For this review, take the finished solid that the model builds, in its own axes (mm). A direction names the side the tool comes from. Coordinates: 2 decimals unless noted, no trailing zeros. Loops run counter-clockwise (first coordinate to the right, second up) from the corner with the lowest first, then second, coordinate; pieces in that order, holes last. Notation, with made-up numbers: M -8,51.5 L 38,51.5 A9 cw 38,67.5 Z; hole C -28,30.25 d8. An arc over 180 degrees is marked long. Put each result on its own line as item: value.
```python
from build123d import *

# Parameters (mm, degrees)
SKETCH1_W               = 50
SKETCH1_H               = 51
BOSS_EXTRUDE1_DEPTH     = 3
SKETCH2_W               = 50
SKETCH2_H               = 3
BOSS_EXTRUDE2_DEPTH     = 50
FILLET1_R               = 2
CHAMFER1_SIZE           = 5
SKETCH4_R               = 12.55
SKETCH4_R_2             = 2.1
CUT_EXTRUDE2_DEPTH      = 50
BOSS_EXTRUDE3_DEPTH     = 3
CROQUIS1_W              = 117.155
CROQUIS1_H              = 77.15
SALIENTE_EXTRUIR1_DEPTH = 10
CROQUIS2_W              = 76.4
CROQUIS2_H              = 56.4
SALIENTE_EXTRUIR2_DEPTH = 7.5
CROQUIS3_R              = 2
CORTAR_EXTRUIR1_DEPTH   = 27.5
CROQUIS4_W              = 91
CROQUIS4_H              = 72
CROQUIS4_W_2            = 79
CROQUIS4_H_2            = 57
SALIENTE_EXTRUIR3_DEPTH = 120
CUT_EXTRUDE1_DEPTH      = 50
CROQUIS5_W              = 66
CROQUIS5_H              = 90
CORTAR_EXTRUIR2_DEPTH   = 64
CROQUIS7_R              = 2.1
CORTAR_EXTRUIR3_DEPTH   = 20
CROQUIS9_R              = 2
CORTAR_EXTRUIR5_DEPTH   = 110
CROQUIS8_R              = 2
CORTAR_EXTRUIR6_DEPTH   = 120
CROQUIS10_R             = 17.5
SALIENTE_EXTRUIR4_DEPTH = 7.5
CROQUIS11_W             = 81
CROQUIS11_H             = 10
CROQUIS11_W_2           = 5
CORTAR_EXTRUIR7_DEPTH   = 7.9
CROQUIS12_W             = 79
CROQUIS12_H             = 4.5
SALIENTE_EXTRUIR5_DEPTH = 12.5
CROQUIS14_W             = 10
CROQUIS14_H             = 3.6
CORTAR_EXTRUIR8_DEPTH   = 100
CROQUIS21_R             = 1.25
CORTAR_EXTRUIR10_DEPTH  = 4
CROQUIS22_R             = 1.5
CORTAR_EXTRUIR11_DEPTH  = 40
CROQUIS23_W             = 10
CROQUIS23_H             = 10
CORTAR_EXTRUIR12_DEPTH  = 10
CROQUIS24_W             = 2
CROQUIS24_H             = 52.5
CORTAR_EXTRUIR13_DEPTH  = 22.5


with BuildPart() as part:
    # Sketch1 → Boss-Extrude1 (new body)
    with BuildSketch(Plane.XY):
        Rectangle(SKETCH1_W, SKETCH1_H)
    extrude(amount=BOSS_EXTRUDE1_DEPTH)

    # Sketch2 → Boss-Extrude2 (add)
    with BuildSketch(Plane.XY.offset(3)):
        with Locations((0, -24)):
            Rectangle(SKETCH2_W, SKETCH2_H)
    extrude(amount=BOSS_EXTRUDE2_DEPTH)

    # Fillet1
    fillet1_edges = [part.edges().sort_by_distance(p)[0] for p in [
        (0, -22.5, 3),
        (0, -25.5, 0),
    ]]
    fillet(fillet1_edges, radius=FILLET1_R)

    # Chamfer1
    chamfer1_edges = [part.edges().sort_by_distance(p)[0] for p in [
        (-25, -24, 53),
        (25, -24, 53),
        (-25, 25.5, 1.5),
        (25, 25.5, 1.5),
    ]]
    chamfer(chamfer1_edges, length=CHAMFER1_SIZE)

    # Sketch4 → Cut-Extrude2 (cut)
    with BuildSketch(Plane.XY.offset(3)):
        with Locations((0, 4.5)):
            Circle(SKETCH4_R)
        with Locations((0, 22)):
            Circle(SKETCH4_R_2)
        with Locations((0, -13)):
            Circle(SKETCH4_R_2)
        with Locations((17.5, 4.5)):
            Circle(SKETCH4_R_2)
        with Locations((-17.5, 4.5)):
            Circle(SKETCH4_R_2)
    extrude(amount=-CUT_EXTRUDE2_DEPTH, mode=Mode.SUBTRACT)

    # Sketch5 → Boss-Extrude3 (add)
    with BuildSketch(Plane.ZY.offset(25)):
        with BuildLine():
            Line((3, -2.5), (16, -22.5))
            Line((16, -22.5), (5, -22.5))
            ThreePointArc((5, -22.5), (3.585786438, -21.914213562), (3, -20.5))
            Line((3, -20.5), (3, -2.5))
        make_face()
    boss_extrude3 = extrude(amount=-BOSS_EXTRUDE3_DEPTH)

    # Mirror1: Boss-Extrude3 across plane
    add(boss_extrude3.mirror(Plane(origin=(0, 0, 0), x_dir=(0, 0, 1), z_dir=(1, 0, 0))))



with BuildPart() as body_2:
    # Croquis1 → Saliente-Extruir1 (new body)
    with BuildSketch(Plane(origin=(0, 0, 55), x_dir=(-1, 0, 0), z_dir=(0, 0, -1))):
        with Locations((0.0025, 0)):
            Rectangle(CROQUIS1_W, CROQUIS1_H)
    extrude(amount=-SALIENTE_EXTRUIR1_DEPTH)

    # Croquis2 → Saliente-Extruir2 (add)
    with BuildSketch(Plane.XY.offset(65)):
        Rectangle(CROQUIS2_W, CROQUIS2_H)
    extrude(amount=SALIENTE_EXTRUIR2_DEPTH)

    # Croquis3 → Cortar-Extruir1 (cut)
    with BuildSketch(Plane(origin=(0, 0, 55), x_dir=(-1, 0, 0), z_dir=(0, 0, -1))):
        with Locations((50.58, -18.575)):
            Circle(CROQUIS3_R)
        with Locations((50.58, 18.575)):
            Circle(CROQUIS3_R)
    cortar_extruir1 = extrude(amount=-CORTAR_EXTRUIR1_DEPTH, mode=Mode.SUBTRACT)

    # Simetría1: Cortar-Extruir1 across plane
    add(cortar_extruir1.mirror(Plane(origin=(0, 0, 0), x_dir=(0, 0, 1), z_dir=(1, 0, 0))), mode=Mode.SUBTRACT)


with BuildPart() as part_1:
    add(part.part)

    add(body_2.part)  # Saliente-Extruir3 merges body 2
    # Croquis4 → Saliente-Extruir3 (add)
    with BuildSketch(Plane(origin=(0, 0, 55), x_dir=(-1, 0, 0), z_dir=(0, 0, -1))):
        with Locations((0.5, 2.5)):
            Rectangle(CROQUIS4_W, CROQUIS4_H)
        with Locations((1.5, 3)):
            Rectangle(CROQUIS4_W_2, CROQUIS4_H_2, mode=Mode.SUBTRACT)
    extrude(amount=SALIENTE_EXTRUIR3_DEPTH)

    # Sketch3 → Cut-Extrude1 (cut)
    with BuildSketch(Plane(origin=(0, -22.5, 0), x_dir=(1, 0, 0), z_dir=(0, 1, 0))):
        with BuildLine():
            Line((-17.1, -38), (-17.1, -37.9))
            ThreePointArc((-17.1, -37.9), (-15, -35.8), (-12.9, -37.9))
            Line((-12.9, -37.9), (-12.9, -38))
            ThreePointArc((-12.9, -38), (-15, -40.1), (-17.1, -38))
        make_face()
        with BuildLine():
            Line((12.9, -38), (12.9, -37.9))
            ThreePointArc((12.9, -37.9), (15, -35.8), (17.1, -37.9))
            Line((17.1, -37.9), (17.1, -38))
            ThreePointArc((17.1, -38), (15, -40.1), (12.9, -38))
        make_face()
    extrude(amount=-CUT_EXTRUDE1_DEPTH, mode=Mode.SUBTRACT)

    # Croquis5 → Cortar-Extruir2 (cut)
    with BuildSketch(Plane(origin=(0, 38.5, 0), x_dir=(1, 0, 0), z_dir=(0, 1, 0))):
        with Locations((-0.5, -10)):
            Rectangle(CROQUIS5_W, CROQUIS5_H)
    extrude(amount=-CORTAR_EXTRUIR2_DEPTH, mode=Mode.SUBTRACT)

    # Croquis7 → Cortar-Extruir3 (cut)
    with BuildSketch(Plane.XZ.offset(33.5)):
        with Locations((15, 19.753839811)):
            Circle(CROQUIS7_R)
        with Locations((-15, 19.753839811)):
            Circle(CROQUIS7_R)
    extrude(amount=-CORTAR_EXTRUIR3_DEPTH, mode=Mode.SUBTRACT)

    # Croquis9 → Cortar-Extruir5 (cut)
    with BuildSketch(Plane.ZY.offset(46)):
        with Locations((-49, -18.5)):
            Circle(CROQUIS9_R)
        with Locations((-49, 5.5)):
            Circle(CROQUIS9_R)
    extrude(amount=-CORTAR_EXTRUIR5_DEPTH, mode=Mode.SUBTRACT)

    # Croquis8 → Cortar-Extruir6 (cut)
    with BuildSketch(Plane(origin=(0, 38.5, 0), x_dir=(1, 0, 0), z_dir=(0, 1, 0))):
        with Locations((-10.5, 49)):
            Circle(CROQUIS8_R)
        with Locations((9.5, 49)):
            Circle(CROQUIS8_R)
    extrude(amount=-CORTAR_EXTRUIR6_DEPTH, mode=Mode.SUBTRACT)

    # Croquis10 → Saliente-Extruir4 (add)
    with BuildSketch(Plane(origin=(0, 0, -35), x_dir=(-1, 0, 0), z_dir=(0, 0, -1))):
        Polygon((41, 0), (41, -25.5), (-40, -25.5), (-40, 31.5), (41, 31.5), align=None)
        with Locations((0, 3)):
            Circle(CROQUIS10_R, mode=Mode.SUBTRACT)
    extrude(amount=SALIENTE_EXTRUIR4_DEPTH)

    # Croquis11 → Cortar-Extruir7 (cut)
    with BuildSketch(Plane(origin=(0, 38.5, 0), x_dir=(1, 0, 0), z_dir=(0, 1, 0))):
        with Locations((-0.5, 60)):
            Rectangle(CROQUIS11_W, CROQUIS11_H)
        with Locations((-43.5, 60)):
            Rectangle(CROQUIS11_W_2, CROQUIS11_H)
        with Locations((42.5, 60)):
            Rectangle(CROQUIS11_W_2, CROQUIS11_H)
    extrude(amount=-CORTAR_EXTRUIR7_DEPTH, mode=Mode.SUBTRACT)

    # Croquis12 → Saliente-Extruir5 (add)
    with BuildSketch(Plane(origin=(0, 0, -42.5), x_dir=(-1, 0, 0), z_dir=(0, 0, -1))):
        with Locations((1.5, 29.25)):
            Rectangle(CROQUIS12_W, CROQUIS12_H)
    extrude(amount=SALIENTE_EXTRUIR5_DEPTH)

    # Croquis14 → Cortar-Extruir8 (cut)
    with BuildSketch(Plane(origin=(45, 0, 0), x_dir=(0, 0, -1), z_dir=(1, 0, 0))):
        with Locations((60, 28.8)):
            Rectangle(CROQUIS14_W, CROQUIS14_H)
    extrude(amount=-CORTAR_EXTRUIR8_DEPTH, mode=Mode.SUBTRACT)

    # Croquis21 → Cortar-Extruir10 (cut)
    with BuildSketch(Plane(origin=(45, 0, 0), x_dir=(0, 0, -1), z_dir=(1, 0, 0))):
        with Locations((-40, 32)):
            Circle(CROQUIS21_R)
        with Locations((-40, 19)):
            Circle(CROQUIS21_R)
    extrude(amount=-CORTAR_EXTRUIR10_DEPTH, mode=Mode.SUBTRACT)

    # Croquis22 → Cortar-Extruir11 (cut)
    with BuildSketch(Plane.XZ.offset(33.5)):
        with Locations((30, -30)):
            Circle(CROQUIS22_R)
        with Locations((30, -20)):
            Circle(CROQUIS22_R)
    extrude(amount=-CORTAR_EXTRUIR11_DEPTH, mode=Mode.SUBTRACT)

    # Croquis23 → Cortar-Extruir12 (cut)
    with BuildSketch(Plane.ZY.offset(46)):
        with Locations((50, 8.5)):
            Rectangle(CROQUIS23_W, CROQUIS23_H)
    extrude(amount=-CORTAR_EXTRUIR12_DEPTH, mode=Mode.SUBTRACT)

    # Croquis24 → Cortar-Extruir13 (cut)
    with BuildSketch(Plane(origin=(0, 0, -65), x_dir=(-1, 0, 0), z_dir=(0, 0, -1))):
        with Locations((-39, 0.75)):
            Rectangle(CROQUIS24_W, CROQUIS24_H)
    extrude(amount=-CORTAR_EXTRUIR13_DEPTH, mode=Mode.SUBTRACT)


solid = part_1.part
```
(1) Add section A-A (z = 48.5). Write out the cut boundary in (x, y), plus the area to 3 significant figures.
Determined:
outline: M -46,-33.5 L 45,-33.5 L 45,38.5 L 32.5,38.5 L 32.5,31.5 L 38,31.5 L 38,-25.5 L -41,-25.5 L -41,3.5 L -46,3.5 Z; M -46,13.5 L -41,13.5 L -41,31.5 L -33.5,31.5 L -33.5,38.5 L -46,38.5 Z
area: 1,540 mm^2
(2) Draft analysis for pull direction Z (two halves, no side actions). For faces 4 (the flat face through (35, 31.5, 11)), 5 (the flat face through (40, 0, -54)), 6 (the flat face through (6, -28, -65)), state which applies: +Z half, -Z half, draft (parallel to the pull), parting line (faces both ways), or undercut.
Determined:
face 4: undercut
face 5: draft
face 6: -Z half
(3) Add section B-B (x = -36.5). Write out the cut boundary in (y, z) (3 decimals), plus the area to 3 significant figures.
Determined:
outline: M -38.575,55 L -33.5,55 L -33.5,-65 L -25.5,-65 L -25.5,-42.5 L 27,-42.5 L 27,-55 L 38.5,-55 L 38.5,55 L 38.575,55 L 38.575,65 L 28.2,65 L 28.2,72.5 L -28.2,72.5 L -28.2,65 L -38.575,65 Z; hole M -25.5,-35 L 31.5,-35 L 31.5,55 L -25.5,55 Z
area: 3,410 mm^2
(4) Tool access review of faces 1 (the flat face through (45, 2, -4)), 2 (the flat face through (-1, -28.2, 69)), 3 (the flat face through (32.5, 35, 11)): name each direction out of +Z, -Z, +X, -X, +Y, -Y from which nothing blocks a thin tool from reaching the whole face with its end or side.
Determined:
face 1: -Z, +X, +Y, -Y
face 2: +Z, +X, -X, -Y
face 3: +Y
(5) Add section D-D (y = 10). Write out the cut boundary in (x, z) (3 decimals), plus the area to 3 significant figures.
Determined:
outline: M -58.58,55 L 38,55 L 38,-35 L 16.039,-35 L 16.039,-42.5 L 40,-42.5 L 40,-65 L 45,-65 L 45,55 L 58.575,55 L 58.575,65 L 38.2,65 L 38.2,72.5 L -38.2,72.5 L -38.2,65 L -58.58,65 Z; M -46,-65 L -41,-65 L -41,-42.5 L -16.039,-42.5 L -16.039,-35 L -41,-35 L -41,45 L -46,45 Z
area: 3,440 mm^2
(6) Wall thickness on line 1 along Y through (x, z) = (43.75, 40); line 2 along X through (y, z) = (-31, -49); line 3 along Y through (x, z) = (50.58, 59.75) (3 decimals): over which ranges is each line inside the solid? List them lowest first. Write a range as [from, to].
Determined:
line 1: y = [-33.5, 17.75], [20.25, 30.75], [33.25, 38.5]
line 2: x = [-46, -12.5], [-8.5, 7.5], [11.5, 45]
line 3: y = [-38.575, -20.575], [-16.575, 16.575], [20.575, 38.575]
(7) For pin 1 (6 mm diameter, centred on x = -33, z = 4.5, fed in from -Y); pin 2 (1 mm diameter, centred on x = -20.5, y = 14.5, fed in from -Z); pin 3 (6 mm diameter, centred on y = 9, z = 70, fed in from -X), all flat-tipped, find the tip position at first contact; note any pin that passes through.
Determined:
pin 1: stops at y = -33.5
pin 2: stops at z = -42.5
pin 3: stops at x = -38.2
(8) Add section C-C (x = 0). Write out the cut boundary in (y, z) (3 decimals), plus the area to 3 significant figures.
Determined:
outline: M -38.575,55 L -33.5,55 L -33.5,-65 L -25.5,-65 L -25.5,-42.5 L -14.5,-42.5 L -14.5,-35 L -25.5,-35 L -25.5,55 L 38.575,55 L 38.575,65 L 28.2,65 L 28.2,72.5 L -28.2,72.5 L -28.2,65 L -38.575,65 Z; M 20.5,-42.5 L 27,-42.5 L 27,-55 L 38.5,-55 L 38.5,-35 L 20.5,-35 Z
area: 2,520 mm^2
